Here's the drawing with two shaded views (mm, measured from the low corner). I have some questions. Round coordinates to 2 decimals unless told otherwise and drop trailing zeros. Order: outer loops, then holes, each group sorted by start corner. A loop starts at its lowest first (then second) coordinate and runs counter-clockwise, first axis right, second up. Notation, with made-up numbers: (10, 84) -> (60, 84) arc R16 ccw to (60, 92) -> close; hole circle Ø3 at (-3.75, 1.5). An arc over 180 degrees is marked (long way). Answer in a Markdown table with one row per item.
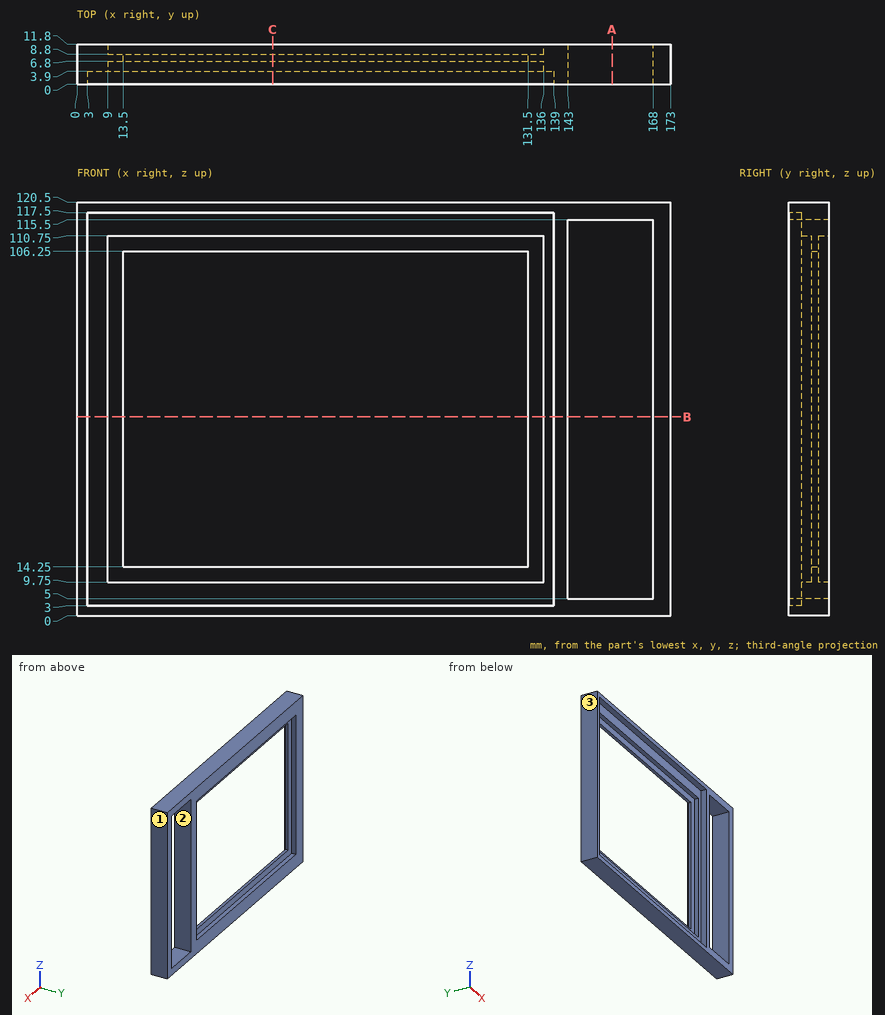
1. Suppose I cut it at C-C on x = 57. Write out the boundary of the cut face in (y, z).
Numbers:
| item | result |
|---|---|
| outline | (0, 0) -> (11.8, 0) -> (11.8, 9.75) -> (8.8, 9.75) -> (8.8, 14.25) -> (6.8, 14.25) -> (6.8, 9.75) -> (3.9, 9.75) -> (3.9, 3) -> (0, 3) -> close; (0, 117.5) -> (3.9, 117.5) -> (3.9, 110.75) -> (6.8, 110.75) -> (6.8, 106.25) -> (8.8, 106.25) -> (8.8, 110.75) -> (11.8, 110.75) -> (11.8, 120.5) -> (0, 120.5) -> close |
2. Suppose I cut it at B-B on z = 58. Write out the boundary of the cut face in (x, y), then the cut area to 3 significant figures.
Numbers:
| item | result |
|---|---|
| outline | (0, 0) -> (3, 0) -> (3, 3.9) -> (9, 3.9) -> (9, 6.8) -> (13.5, 6.8) -> (13.5, 8.8) -> (9, 8.8) -> (9, 11.8) -> (0, 11.8) -> close; (131.5, 6.8) -> (136, 6.8) -> (136, 3.9) -> (139, 3.9) -> (139, 0) -> (143, 0) -> (143, 11.8) -> (136, 11.8) -> (136, 8.8) -> (131.5, 8.8) -> close; (168, 0) -> (173, 0) -> (173, 11.8) -> (168, 11.8) -> close |
| area | 231 mm2 |
3. Suppose I cut it at A-A on x = 156. Write out the boundary of the cut face in (y, z), then the cut area to 3 significant figures.
Numbers:
| item | result |
|---|---|
| outline | (0, 0) -> (11.8, 0) -> (11.8, 5) -> (0, 5) -> close; (0, 115.5) -> (11.8, 115.5) -> (11.8, 120.5) -> (0, 120.5) -> close |
| area | 118 mm2 |
4. We'd pull the mould along X, two halves only. Please class the marked faces 1, 2 and 3: released by +X, released by -X, zero draft, split by the parting line, or undercut.
Numbers:
| item | result |
|---|---|
| face 1 | released by +X |
| face 2 | undercut |
| face 3 | released by -X |
5. Please list where these lines run through material, in increasing order: line 1 along X through (y, z) = (2.5, 34.5); line 2 along X through (y, z) = (8.5, 54.5); line 3 along Z through (x, y) = (66.5, 3.75).
Numbers:
| item | result |
|---|---|
| line 1 | x = 0 to 3, 139 to 143, 168 to 173 |
| line 2 | x = 0 to 13.5, 131.5 to 143, 168 to 173 |
| line 3 | z = 0 to 3, 117.5 to 120.5 |
